Part print with two shaded views. Sizes in mm from the minimum x, y, z corner. Round coordinates to 2 decimals unless told otherwise and drop trailing zeros. Order: outer loops, then holes, each group sorted by start corner. A loop starts at its lowest first (then second) coordinate and runs counter-clockwise, first axis right, second up. Notation, with made-up numbers: (24.5, 55.5) -> (74.5, 55.5) arc R30 cw to (74.5, 79.5) -> close; hole circle Ø4 at (-12, 67). An arc over 180 degrees is marked (long way). Use a Markdown table: item, result. Add a question column.
Item 1: Slice it at C-C, the plane y = 16. Give the cut face in (x, z).
Item 2: Probe L1, parallel to X at y = 22, z = 4 (1 decimal); L2, parallel to X at y = 18.5, z = 2; L3, parallel to Y at x = 26.5, z = 1.75 (1 decimal). List the from-to ranges inside material, lowest first.
Item 3: Two-plate mould, pull along Y, no slides. Class the marked faces 1, 2, 3 and 4: released by +Y, released by -Y, zero draft, split by the parting line, or undercut.
Item 4: Slice it at B-B, the plane z = 6.75. Give the cut face in (x, y), plus the area to 3 significant figures.
Item 5: Slice it at A-A, the plane x = 22.5. Give the cut face in (y, z), plus the area to 3 significant figures.
Item 6: Pin check, flat tips, straight feed: pin 1 (1 mm diameter, centred on y = 19.5, z = 1.5, fed in from -X); pin 2 (3 mm diameter, centred on x = 25, z = 6, fed in from -Y); pin 3 (5 mm diameter, centred on x = 24.5, y = 26, fed in from +Z). Stop position of each tip, or through.
Item 7: Slice it at D-D, the plane x = 16. Give the cut face in (y, z), plus the area to 3 significant figures.
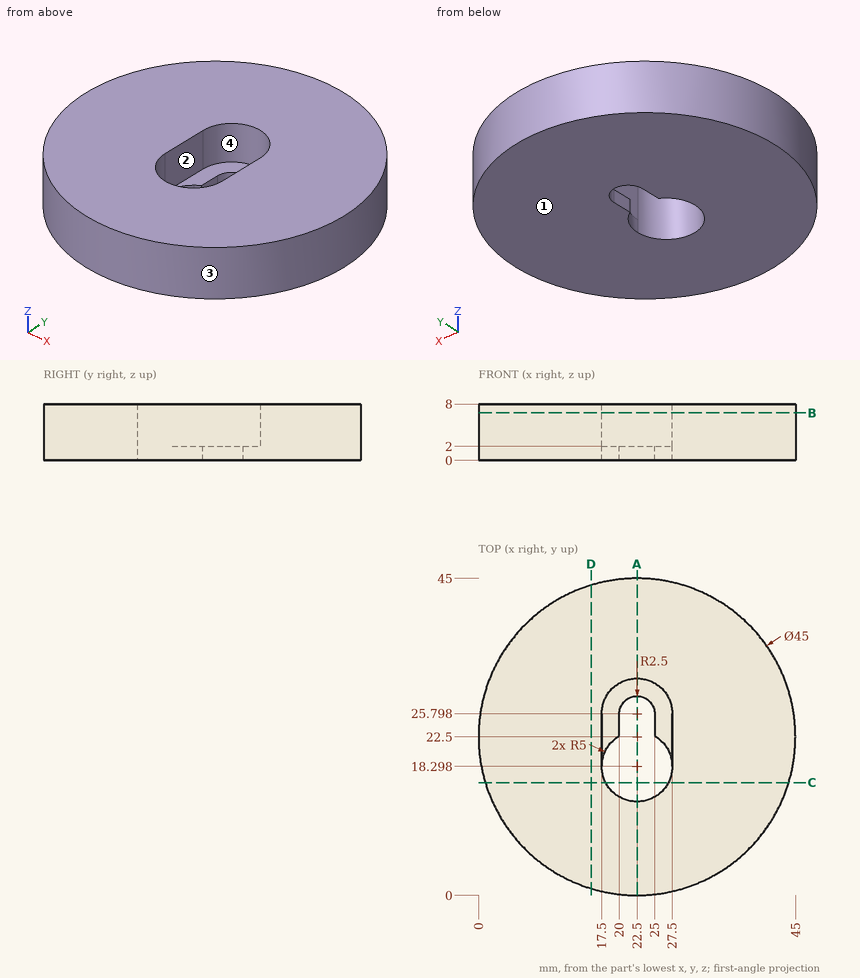
Check sheet entries:
| question | item | result |
|---|---|---|
| 1 | outline | (0.96, 0) -> (18.06, 0) -> (18.06, 8) -> (0.96, 8) -> close; (26.94, 0) -> (44.04, 0) -> (44.04, 8) -> (26.94, 8) -> close |
| 2 | L1 | 0 to 17.5, 27.5 to 45 |
| 2 | L2 | 0.36 to 17.5, 27.5 to 44.64 |
| 2 | L3 | 0.4 to 15.3, 21.3 to 44.6 |
| 3 | face 1 | zero draft |
| 3 | face 2 | undercut |
| 3 | face 3 | split by the parting line |
| 3 | face 4 | undercut |
| 4 | outline | circle Ø45 at (22.5, 22.5); hole (17.5, 18.3) arc R5 ccw to (27.5, 18.3) -> (27.5, 25.8) arc R5 ccw to (17.5, 25.8) -> close |
| 4 | area | 1,440 mm2 |
| 5 | outline | (0, 0) -> (13.3, 0) -> (13.3, 8) -> (0, 8) -> close; (28.3, 0) -> (45, 0) -> (45, 8) -> (30.8, 8) -> (30.8, 2) -> (28.3, 2) -> close |
| 5 | area | 225 mm2 |
| 6 | pin 1 | x = 0.14 |
| 6 | pin 2 | y = 0.02 |
| 6 | pin 3 | z = 2 |
| 7 | outline | (0.96, 0) -> (44.04, 0) -> (44.04, 8) -> (0.96, 8) -> close |
| 7 | area | 345 mm2 |
